Print and shaded views of the part. All mm, measured from the part's lowest x, y and z. Coordinates: 2 decimals unless noted, no trailing zeros. Order: outer loops, then holes, each group sorted by start corner. A loop starts at its lowest first (then second) coordinate and runs counter-clockwise, first axis right, second up. Notation, with made-up numbers: M -26,69.25 L 9,69.25 A30 ccw 9,108.25 Z; hole C 73,-9 d1. An arc over 180 degrees is marked long. Return JSON: item names as keys, results as strings.
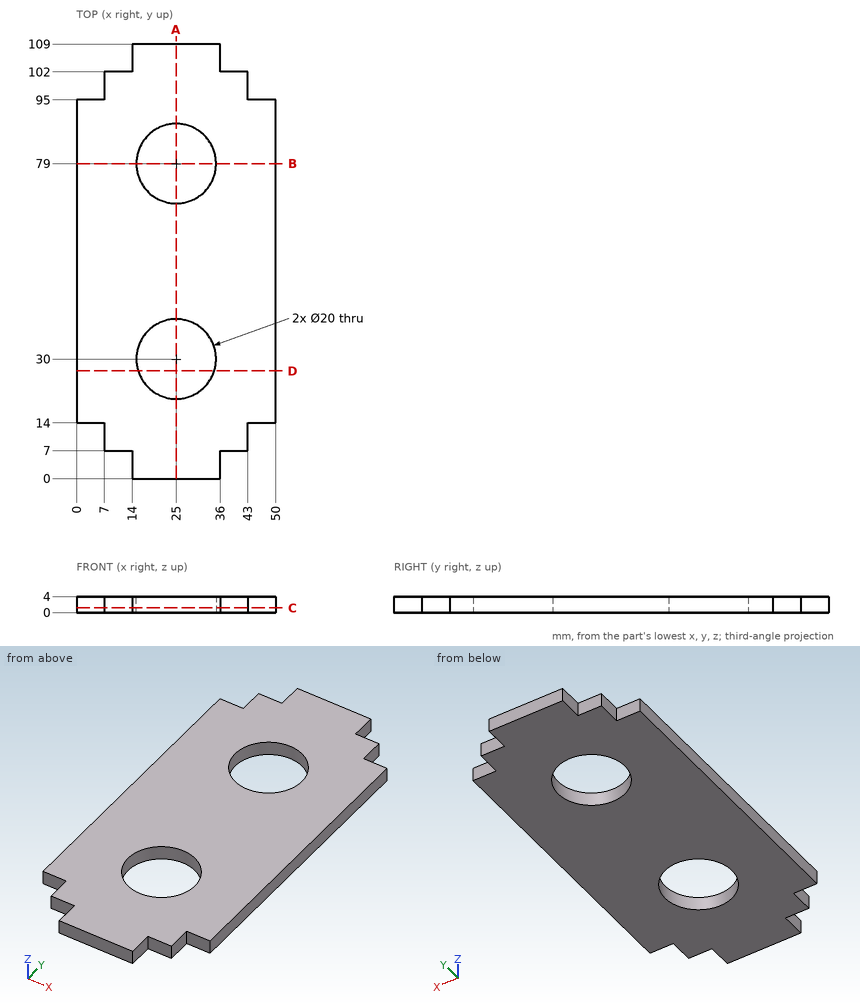
Item 1: Saw through at A-A (x = 25). Write the cut outline in (y, z).
Check result:
{"outline": "M 0,0 L 20,0 L 20,4 L 0,4 Z; M 40,0 L 69,0 L 69,4 L 40,4 Z; M 89,0 L 109,0 L 109,4 L 89,4 Z"}
Item 2: Wall check: line 1 (Y direction, x = 25, z = 2.3); line 2 (Y direction, x = 33, z = 0.25); line 3 (X direction, y = 98, z = 0.7). Give the ranges that are in metal, low to high.
Check result:
{"line 1": "y = 0 to 20, 40 to 69, 89 to 109", "line 2": "y = 0 to 24, 36 to 73, 85 to 109", "line 3": "x = 7 to 43"}
Item 3: Drop flat-ended pins along their axis: pin 1 Ø2 at (x, z) = (40.5, 1.5) entering from +Y; pin 2 Ø1.2 at (y, z) = (3.5, 2.5) entering from +X; pin 3 Ø1.2 at (y, z) = (2.5, 2) entering from -X. Give the stop position or say it passes through.
Check result:
{"pin 1": "stops at y = 102", "pin 2": "stops at x = 36", "pin 3": "stops at x = 14"}
Item 4: Saw through at C-C (z = 1.15). Write the cut outline in (x, y).
Check result:
{"outline": "M 0,14 L 7,14 L 7,7 L 14,7 L 14,0 L 36,0 L 36,7 L 43,7 L 43,14 L 50,14 L 50,95 L 43,95 L 43,102 L 36,102 L 36,109 L 14,109 L 14,102 L 7,102 L 7,95 L 0,95 Z; hole C 25,30 d20; hole C 25,79 d20"}
Item 5: Saw through at D-D (y = 27). Write the cut outline in (x, z).
Check result:
{"outline": "M 0,0 L 15.46,0 L 15.46,4 L 0,4 Z; M 34.54,0 L 50,0 L 50,4 L 34.54,4 Z"}
Item 6: Saw through at B-B (y = 79). Write the cut outline in (x, z).
Check result:
{"outline": "M 0,0 L 15,0 L 15,4 L 0,4 Z; M 35,0 L 50,0 L 50,4 L 35,4 Z"}
